Part model, mm, in its own coordinate system. A direction names the side the tool comes from. Give positions to 0.01 mm unless a question says otherwise; leave off trailing zeros. Write each loop counter-clockwise with the first axis right and the second up, starting at its lowest first coordinate (ties: lowest second). Pieces come first, ordered by that corner, then holes. Notation, with made-up numbers: M 28.5,4.25 L 43.5,4.25 A21 cw 43.5,31.25 Z; hole C 58,24.5 d11. An arc over 180 degrees is marked long. Use a Markdown table: item, result.
```python
from build123d import *

# Parameters (mm, degrees)
SKETCH1_W           = 45
SKETCH1_H           = 50
BOSS_EXTRUDE1_DEPTH = 5
CUT_EXTRUDE1_DEPTH  = 5
SKETCH6_W           = 5
SKETCH6_H           = 20
BOSS_EXTRUDE2_DEPTH = 5
SKETCH7_W           = 15
SKETCH7_H           = 5
CUT_EXTRUDE2_DEPTH  = 10
CUT_EXTRUDE3_DEPTH  = 5


with BuildPart() as part:
    # Sketch1 → Boss-Extrude1 (new body)
    with BuildSketch(Plane.XY):
        with Locations((-7.5, 0)):
            Rectangle(SKETCH1_W, SKETCH1_H)
    extrude(amount=BOSS_EXTRUDE1_DEPTH)

    # Sketch5 → Cut-Extrude1 (cut)
    with BuildSketch(Plane.XY.offset(5)):
        Polygon((-30, 15.6), (-30, 19.6), (-27, 19.6), (-27, 21.1), (-23.8, 21.1), (-23.8, 19.6), (-18.8, 19.6), (-18.8, 15.6), (-23.8, 15.6), (-23.8, 14.1), (-27, 14.1), (-27, 15.6), align=None)
        Polygon((15, 19.6), (12, 19.6), (12, 21.1), (8.8, 21.1), (8.8, 19.6), (3.8, 19.6), (3.8, 15.6), (8.8, 15.6), (8.8, 14.1), (12, 14.1), (12, 15.6), (15, 15.6), align=None)
    extrude(amount=-CUT_EXTRUDE1_DEPTH, mode=Mode.SUBTRACT)

    # Sketch6 → Boss-Extrude2 (add)
    with BuildSketch(Plane(origin=(0, 0, 0), x_dir=(-1, 0, 0), z_dir=(0, 0, -1))):
        with Locations((-17.5, -15)):
            Rectangle(SKETCH6_W, SKETCH6_H)
        with Locations((32.5, -15)):
            Rectangle(SKETCH6_W, SKETCH6_H)
    extrude(amount=-BOSS_EXTRUDE2_DEPTH)

    # Sketch7 → Cut-Extrude2 (cut)
    with BuildSketch(Plane.XY.offset(5)):
        with Locations((-7.5, 22.5)):
            Rectangle(SKETCH7_W, SKETCH7_H)
    extrude(amount=-CUT_EXTRUDE2_DEPTH, mode=Mode.SUBTRACT)

    # Sketch8 → Cut-Extrude3 (cut)
    with BuildSketch(Plane.XY.offset(5)):
        Polygon((-9.894748858, 20), (-9.894748858, 15), (-11.394748858, 15), (-11.394748858, 11.8), (-9.894748858, 11.8), (-9.894748858, 10), (-5.894748858, 10), (-5.894748858, 11.8), (-4.394748858, 11.8), (-4.394748858, 15), (-5.894748858, 15), (-5.894748858, 20), align=None)
    extrude(amount=-CUT_EXTRUDE3_DEPTH, mode=Mode.SUBTRACT)


solid = part.part
```
1. Drill centre lines: L1, parallel to Y at x = -21.5, z = 3.6; L2, parallel to Y at x = -25, z = 1.9; L3, parallel to X at y = 18, z = 1.3. Where is each one in solid material? Low to high.
Findings below:
| item | result |
|---|---|
| L1 | -25 to 15.6, 19.6 to 25 |
| L2 | -25 to 14.1, 21.1 to 25 |
| L3 | -18.8 to -9.89, -5.89 to 3.8 |
2. Cut at C-C, the plane y = 2.5. Give the cut face in (x, z), then the cut area to 3 significant figures.
Findings below:
| item | result |
|---|---|
| outline | M -30,0 L 15,0 L 15,5 L -30,5 Z |
| area | 225 mm2 |
3. Cut at D-D, the plane x = -12.5. Give the cut face in (y, z), then the cut area to 3 significant figures.
Findings below:
| item | result |
|---|---|
| outline | M -25,0 L 20,0 L 20,5 L -25,5 Z |
| area | 225 mm2 |
4. Cut at B-B, the plane x = -21.5. Give the cut face in (y, z).
Findings below:
| item | result |
|---|---|
| outline | M -25,0 L 15.6,0 L 15.6,5 L -25,5 Z; M 19.6,0 L 25,0 L 25,5 L 19.6,5 Z |
5. Tool access for faces 1 (the flat face through (14, 19.6, 3)), 2 (the flat face through (-3, 20, 3)), 3 (the flat face through (12, 15, 3)), 4 (the flat face through (-32, -5, 2)), 5 (the flat face through (15, 22, 2)): list every direction of +Z, -Z, +X, -X, +Y, -Y with a clear straight run to the whole face (end or side of a thin tool).
Findings below:
| item | result |
|---|---|
| face 1 | +Z, -Z, +X |
| face 2 | +Z, -Z, +Y |
| face 3 | +Z, -Z |
| face 4 | +Z, -Z, -X, +Y |
| face 5 | +Z, -Z, +X, +Y |
6. Cut at A-A, the plane y = 13. Give the cut face in (x, z).
Findings below:
| item | result |
|---|---|
| outline | M -30,0 L -11.39,0 L -11.39,5 L -30,5 Z; M -4.39,0 L 15,0 L 15,5 L -4.39,5 Z |
7. Drop flat-ended pins along their axis: P1, Ø1.2, axis at y = 20.5, z = 2, coming from the +X side; P2, Ø1.6, axis at y = 15, z = 3.5, coming from the -X side; P3, Ø2, axis at x = -8.5, z = 1.5, coming from the +Y side; P4, Ø4, axis at x = -23.5, y = 10.5, coming from the -Z side. Give the stop position or say it passes through.
Findings below:
| item | result |
|---|---|
| P1 | x = 15 |
| P2 | x = -30 |
| P3 | y = 10 |
| P4 | z = 0 |
8. Two-plate mould, pull along X, no slides. Class faces 6 (the flat face through (-9.895, 18, 3)), 7 (the flat face through (20, -15, 2)), 8 (the flat face through (-11.395, 13, 3)), 9 (the flat face through (-28, 15.6, 3)): released by +X, released by -X, zero draft, split by the parting line, or undercut.
Findings below:
| item | result |
|---|---|
| face 6 | undercut |
| face 7 | released by +X |
| face 8 | undercut |
| face 9 | zero draft |
